Read the model definition and answer for the solid it produces. Units are mm, in the model's axes. A direction names the side the tool comes from. Give positions to 0.01 mm unless a question says otherwise; leave off trailing zeros. Order: outer loops, then holes, each group sorted by start corner. A loop starts at its lowest first (then second) coordinate and runs counter-clockwise, first axis right, second up. Notation, with made-up numbers: (73, 49) - (110, 49) arc R31 ccw to (110, 87) - close; hole circle Ø8 at (-15, 1). An arc over 180 degrees is marked (long way). Write item = value, one per line.
```python
from build123d import *

# Parameters (mm, degrees)
ESQUISSE1_W             = 63
ESQUISSE1_H             = 75
BOSS_EXTRU_1_DEPTH      = 900
ESQUISSE2_W             = 63
ESQUISSE2_H             = 75
ENL_V_MAT_EXTRU_1_DEPTH = 19
ENL_V_START             = -63
ESQUISSE2_2_W           = 63
ESQUISSE2_2_H           = 75
ENL_V_MAT_EXTRU_2_DEPTH = 19
ESQUISSE3_R             = 10
ENL_V_MAT_EXTRU_3_DEPTH = 906.31431006


with BuildPart() as part:
    # Esquisse1 → Boss.-Extru.1 (new body)
    with BuildSketch(Plane.XY):
        with Locations((31.5, 37.5)):
            Rectangle(ESQUISSE1_W, ESQUISSE1_H)
    extrude(amount=BOSS_EXTRU_1_DEPTH)

    # Esquisse2 → Enlèv. mat.-Extru.1 (cut)
    with BuildSketch(Plane(origin=(63, 0, 0), x_dir=(0, 0, -1), z_dir=(1, 0, 0))):
        with Locations((-788.5, 37.5)):
            Rectangle(ESQUISSE2_W, ESQUISSE2_H)
        with Locations((-111.5, 37.5)):
            Rectangle(ESQUISSE2_W, ESQUISSE2_H)
    extrude(amount=-ENL_V_MAT_EXTRU_1_DEPTH, mode=Mode.SUBTRACT)

    # Esquisse2<2> → Enlèv. mat.-Extru.2 (cut)
    with BuildSketch(Plane(origin=(63, 0, 0), x_dir=(0, 0, -1), z_dir=(1, 0, 0)).offset(ENL_V_START)):
        with Locations((-788.5, 37.5)):
            Rectangle(ESQUISSE2_2_W, ESQUISSE2_2_H)
        with Locations((-111.5, 37.5)):
            Rectangle(ESQUISSE2_2_W, ESQUISSE2_2_H)
    extrude(amount=ENL_V_MAT_EXTRU_2_DEPTH, mode=Mode.SUBTRACT)

    # Esquisse3 → Enlèv. mat.-Extru.3 (cut, through all)
    with BuildSketch(Plane(origin=(0, 75, 0), x_dir=(1, 0, 0), z_dir=(0, 1, 0))):
        with Locations(Location((31.5, -300, 0), (0, 0, 270))):
            Circle(ESQUISSE3_R)
        with Locations(Location((31.5, -600, 0), (0, 0, 90))):
            Circle(ESQUISSE3_R)
    extrude(amount=-ENL_V_MAT_EXTRU_3_DEPTH, mode=Mode.SUBTRACT)


solid = part.part
```
1. For faces 1 (the face through (9, 37, 143)), 2 (the face through (35.33, 38.025, 590.763)), 3 (the face through (54, 37, 757)), determine the directions among +Z, -Z, +X, -X, +Y, -Y from which every point of the face is accessible in a straight line to the end or side of a thin tool.
Recorded:
face_1 = -X, +Y, -Y
face_2 = +Y, -Y
face_3 = +X, +Y, -Y
2. Section C-C (y = 31.5) is taken. Determine the outline of the cut face in (x, z), and give its area (3 significant figures).
Recorded:
outline = (0, 0) - (63, 0) - (63, 80) - (44, 80) - (44, 143) - (63, 143) - (63, 757) - (44, 757) - (44, 820) - (63, 820) - (63, 900) - (0, 900) - (0, 820) - (19, 820) - (19, 757) - (0, 757) - (0, 143) - (19, 143) - (19, 80) - (0, 80) - close; hole circle Ø20 at (31.5, 300); hole circle Ø20 at (31.5, 600)
area = 51,300 mm^2
3. Section B-B (z = 600) is taken. Determine the outline of the cut face in (x, y), and give its area (4 significant figures).
Recorded:
outline = (0, 0) - (21.5, 0) - (21.5, 75) - (0, 75) - close; (41.5, 0) - (63, 0) - (63, 75) - (41.5, 75) - close
area = 3,225 mm^2
4. Flat-ended cylindrical pins translate along their axes: pin 1 (19 mm diameter, centred on y = 29.5, z = 102, fed in from -X); pin 2 (18 mm diameter, centred on x = 31.5, z = 300, fed in from -Y). Find the tip coordinate at first contact, or state that the pin passes through.
Recorded:
pin_1 = 19
pin_2 = through
5. Section A-A (x = 31.5) is taken. Determine the outline of the cut face in (y, z).
Recorded:
outline = (0, 0) - (75, 0) - (75, 290) - (0, 290) - close; (0, 310) - (75, 310) - (75, 590) - (0, 590) - close; (0, 610) - (75, 610) - (75, 900) - (0, 900) - close
6. Determine the mould class of faces 4 (the face through (31, 38, 900)), 5 (the face through (44, 38, 789)), 6 (the face through (63, 37, 39)) for opening direction Z: +Z half, -Z half, draft (parallel to the pull), parting line (faces both ways), or undercut.
Recorded:
face_4 = +Z half
face_5 = undercut
face_6 = draft
7. Straight lines are drawn through the part: L1, parallel to Z at x = 46, y = 70.5; L2, parallel to Z at x = 31, y = 26; L3, parallel to X at y = 22, z = 300. For each, find the intervals that lie inside material, in ascending order. Write a range as [from, to].
Recorded:
L1 = [0, 80], [143, 757], [820, 900]
L2 = [0, 290.01], [309.99, 590.01], [609.99, 900]
L3 = [0, 21.5], [41.5, 63]
8. Section D-D (z = 130.5) is taken. Determine the outline of the cut face in (x, y), and give its area (4 significant figures).
Recorded:
outline = (19, 0) - (44, 0) - (44, 75) - (19, 75) - close
area = 1,875 mm^2
